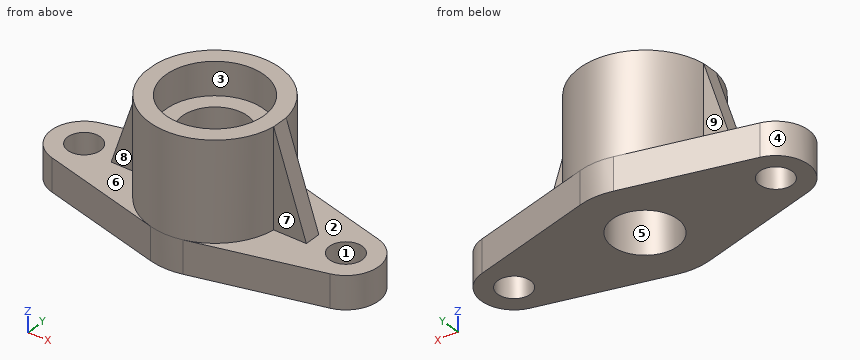
from build123d import *

# Parameters (mm, degrees)
F1_DEPTH  = 10
F2_R      = 5
F3_DEPTH  = 10.001
F4_R      = 20
F5_DEPTH  = 30
F6_R      = 15
F7_DEPTH  = 10
F8_R      = 10
F9_DEPTH  = 30.001
F12_DEPTH = 30
F14_DEPTH = 22.501


with BuildPart() as f1:
    # F0 (on Top) → F1 (new body)
    with BuildSketch(Plane.XY):
        with BuildLine():
            Line((-42.4998887826, -9.6824870811), (-5.0000000003, -19.364916731))
            ThreePointArc((-5.0000000003, -19.364916731), (0, -20), (5.0000000003, -19.364916731))
            Line((5.0000000003, -19.364916731), (42.4998887826, -9.6824870811))
            ThreePointArc((42.4998887826, -9.6824870811), (50, 0), (42.4998887826, 9.6824870811))
            Line((42.4998887826, 9.6824870811), (5.128827219, 19.3311958077))
            ThreePointArc((5.128827219, 19.3311958077), (0, 20), (-5.128827219, 19.3311958077))
            Line((-5.128827219, 19.3311958077), (-42.4998887826, 9.6824870811))
            ThreePointArc((-42.4998887826, 9.6824870811), (-50, 0), (-42.4998887826, -9.6824870811))
        make_face()
    extrude(amount=F1_DEPTH)

    # F2 (on face) → F3 (cut, through all)
    with BuildSketch(Plane.XY.offset(10)):
        with Locations((-40, 0)):
            Circle(F2_R)
        with Locations((40, 0)):
            Circle(F2_R)
    extrude(amount=-F3_DEPTH, mode=Mode.SUBTRACT)

    # F4 (on face) → F5 (join)
    with BuildSketch(Plane.XY.offset(10)):
        Circle(F4_R)
    extrude(amount=F5_DEPTH)

    # F6 (on face) → F7 (cut)
    with BuildSketch(Plane.XY.offset(40)):
        Circle(F6_R)
    extrude(amount=-F7_DEPTH, mode=Mode.SUBTRACT)

    # F8 (on face) → F9 (cut, through all)
    with BuildSketch(Plane.XY.offset(30)):
        Circle(F8_R)
    extrude(amount=-F9_DEPTH, mode=Mode.SUBTRACT)

    # F11 (on offset) → F12 (join)
    with BuildSketch(Plane.XY.offset(10)):
        Polygon((-19.8240634054, -2.5), (-19.8240634054, 0), (-19.8240634054, 2.5), (-29.8240634054, 2.5), (-29.8240634054, 0), (-29.8240634054, -2.5), align=None)
        Polygon((29.8240634054, 2.5), (19.8240634054, 2.5), (19.8240634054, 0), (19.8240634054, -2.5), (29.8240634054, -2.5), (29.8240634054, 0), align=None)
    extrude(amount=F12_DEPTH)

    # F13 (on face) → F14 (cut, through all)
    with BuildSketch(Plane.XZ.offset(2.5)):
        Polygon((-29.8240634054, 40), (-29.8240634054, 10), (-19.843134833, 40), align=None)
        Polygon((19.843134833, 40), (29.8240634054, 10), (29.8240634054, 40), align=None)
    extrude(amount=-F14_DEPTH, mode=Mode.SUBTRACT)


solid = f1.part
Verification items for the finished model (mm, model axes). Face numbers are marked on the shaded views. A direction names the side the tool comes from. Give positions to 0.01 mm unless a question says otherwise; leave off trailing zeros. Loops run counter-clockwise (first coordinate to the right, second up) from the corner with the lowest first, then second, coordinate; pieces in that order, holes last.
1. Cross-section at A-A on y = 0. Record the cut outline in (x, z), and give its area (3 significant figures).
Derived:
outline: (-50, 0) - (-45, 0) - (-45, 10) - (-50, 10) - close; (-35, 0) - (-10, 0) - (-10, 30) - (-15, 30) - (-15, 40) - (-19.84, 40) - (-29.82, 10) - (-35, 10) - close; (10, 0) - (35, 0) - (35, 10) - (29.82, 10) - (19.84, 40) - (15, 40) - (15, 30) - (10, 30) - close; (45, 0) - (50, 0) - (50, 10) - (45, 10) - close
area: 1,390 mm2
2. Cross-section at C-C on z = 5. Record the cut outline in (x, y), and give its area (3 significant figures).
Derived:
outline: (-42.5, -9.68) - (-5, -19.36) arc R20 ccw to (5, -19.36) - (42.5, -9.68) arc R10 ccw to (42.5, 9.68) - (5.13, 19.33) arc R20 ccw to (-5.13, 19.33) - (-42.5, 9.68) arc R10 ccw to start; hole circle Ø10 at (-40, 0); hole circle Ø20 at (0, 0); hole circle Ø10 at (40, 0)
area: 2,320 mm2
3. Release check for a two-part mould opening along X. For the marked faces 1, 2, 3 and 4 record: +X half, -X half, draft (parallel to the pull), parting line (faces both ways), or undercut.
Derived:
face 1: undercut
face 2: draft
face 3: undercut
face 4: -X half
4. Material ranges on probe 1 along Y at (x, z) = (0, 35.75); probe 2 along Y at (x, z) = (40, 8); probe 3 along X at (y, z) = (-4.5, 11.5), recorded low to high.
Derived:
probe 1: y = -20 to -15, 15 to 20
probe 2: y = -10.33 to -5, 5 to 10.33
probe 3: x = -19.49 to -8.93, 8.93 to 19.49
5. Cross-section at B-B on x = 0. Record the cut outline in (y, z), and give its area (3 significant figures).
Derived:
outline: (-20, 0) - (-10, 0) - (-10, 30) - (-15, 30) - (-15, 40) - (-20, 40) - close; (10, 0) - (20, 0) - (20, 40) - (15, 40) - (15, 30) - (10, 30) - close
area: 700 mm2
6. Tool access check on the marked faces 5, 6, 7, 8 and 9. Record the directions out of +Z, -Z, +X, -X, +Y, -Y that give a thin tool (end or side, any length) a straight path to the whole face; none if there is none.
Derived:
face 5: +Z, -Z
face 6: +Z, -X
face 7: +Z, +X, -Y
face 8: +Z, -X, -Y
face 9: +Z, -X, +Y
7. Go/stop test with flat-tipped pins: P1, Ø4, axis at y = -8, z = 11.5, coming from the +X side; P2, Ø10, axis at x = 33, y = 0, coming from the -Z side; P3, Ø5, axis at x = 23, z = 30, coming from the -Y side; P4, Ø1, axis at x = 2.5, y = 10, coming from the +Z side. Record where each tip stops, or that it passes through.
Derived:
P1: stops at x = 47.44
P2: stops at z = 0
P3: stops at y = -2.5
P4: stops at z = 30
8. Cross-section at D-D on y = -8. Record the cut outline in (x, z).
Derived:
outline: (-46, 0) - (-6, 0) - (-6, 30) - (-12.69, 30) - (-12.69, 40) - (-18.33, 40) - (-18.33, 10) - (-46, 10) - close; (6, 0) - (46, 0) - (46, 10) - (18.33, 10) - (18.33, 40) - (12.69, 40) - (12.69, 30) - (6, 30) - close
